Geometry check sheet. Reference: the model listing, model coordinates, mm. A direction names the side the tool comes from. Give positions to 0.01 mm unless a question says otherwise; leave off trailing zeros. Write each loop counter-clockwise with the first axis right and the second up, starting at its lowest first coordinate (ties: lowest second). Pieces come first, ordered by that corner, then holes. Notation, with made-up numbers: (58.25, -18.75) - (75.25, -18.75) arc R33 cw to (75.25, 19.25) - close; hole circle Ø1 at (-14.75, 24.5). An arc over 180 degrees is marked (long way). Write item = value, one per line. Start each with the question number.
(1) Thickness scan on L1, parallel to X at y = -45.5, z = 22; L2, parallel to Y at x = 25, z = 57. Record the ranges inside material, lowest first.
(2) Section check D-D, the plane z = 53. Enter the section's corners in (x, y), plus the area to 3 significant figures.
(3) Section check B-B, the plane x = -56. Enter the section's corners in (y, z).
(4) Depth check by flat-ended pin: pin 1 Ø12 at (x, y) = (14.5, -46.5) entering from -Z; pin 2 Ø5.5 at (y, z) = (-15.96, 19.23) entering from -X; pin 3 Ø6.5 at (x, z) = (33.28, 79.04) entering from +Y. Enter the tip coordinate at first touch or a pass-through.
(5) Draft check along Y on faces 1 (the flat face through (-5, -51.506, 41)), 2 (the cylindrical face through (60.6, -16.47, 61.35)), 3 (the flat face through (63.102, -26, 41)). Enter one of: pulls with the +Y half, pulls with the -Y half, needs draft (parallel to the pull), parting line crosses it, or undercut.
(6) Section check A-A, the plane z = 35. Enter the section's corners in (x, y).
(7) Section check C-C, the plane y = -23. Enter the section's corners in (x, z), plus the area to 3 significant figures.
(8) Access from +Z, -Z, +X, -X, +Y, -Y to the whole of each face (thin tool, end or side, straight path). Record for faces 4 (the flat face through (58.022, -4, 41)), 5 (the flat face through (-68.978, -54, 41)).
```python
from build123d import *

# Parameters (mm, degrees)
F1_DEPTH = 82.55
F3_D     = 19.05
F4_D     = 4.7752
F5_D     = 4.7752
F7_D     = 5.08


with BuildPart() as f1:
    # F0 (on Top) → F1 (new body)
    with BuildSketch(Plane.XY):
        Polygon((58.022249, -51.505502), (-68.977751, -51.505502), (-68.977751, -56.585502), (63.102249, -56.585502), (63.102249, 24.694498), (58.022249, 24.694498), align=None)
    extrude(amount=F1_DEPTH)

    # F3 (through all)
    with Locations(Plane(origin=(58.022249, 0, 0), x_dir=(0, -1, 0), z_dir=(-1, 0, 0))):
        with Locations((15.955091, 41.455898)):
            Hole(F3_D / 2)

    # F4 (through all)
    with Locations(Plane(origin=(58.022249, 0, 0), x_dir=(0, -1, 0), z_dir=(-1, 0, 0))):
        with Locations((15.955091, 63.680898)):
            Hole(F4_D / 2)

    # F5 (through all)
    with Locations(Plane(origin=(58.022249, 0, 0), x_dir=(0, -1, 0), z_dir=(-1, 0, 0))):
        with Locations((15.955091, 19.230898)):
            Hole(F5_D / 2)

    # F7 (through all)
    with Locations(Plane(origin=(0, -51.505502, 0), x_dir=(-1, 0, 0), z_dir=(0, 1, 0))):
        with Locations((-33.277512, 79.039508), (54.963514, 79.039508), (54.963514, 3.499908), (-33.277512, 3.499908)):
            Hole(F7_D / 2)


solid = f1.part
```
Model answer:
q1.L1 = 58.02 to 63.1
q1.L2 = -56.59 to -51.51
q2.outline = (-68.98, -56.59) - (63.1, -56.59) - (63.1, 24.69) - (58.02, 24.69) - (58.02, -51.51) - (-68.98, -51.51) - close
q2.area = 1,060 mm²
q3.outline = (-56.59, 0) - (-51.51, 0) - (-51.51, 1.18) - (-56.59, 1.18) - close; (-56.59, 5.82) - (-51.51, 5.82) - (-51.51, 76.72) - (-56.59, 76.72) - close; (-56.59, 81.36) - (-51.51, 81.36) - (-51.51, 82.55) - (-56.59, 82.55) - close
q4.pin_1 = 0
q4.pin_2 = 58.02
q4.pin_3 = -51.51
q5.face_1 = pulls with the +Y half
q5.face_2 = undercut
q5.face_3 = needs draft
q6.outline = (-68.98, -56.59) - (63.1, -56.59) - (63.1, -22.96) - (58.02, -22.96) - (58.02, -51.51) - (-68.98, -51.51) - close; (58.02, -8.95) - (63.1, -8.95) - (63.1, 24.69) - (58.02, 24.69) - close
q7.outline = (58.02, 0) - (63.1, 0) - (63.1, 35.05) - (58.02, 35.05) - close; (58.02, 47.87) - (63.1, 47.87) - (63.1, 82.55) - (58.02, 82.55) - close
q7.area = 354 mm²
q8.face_4 = +Z, -Z, -X, +Y
q8.face_5 = +Z, -Z, -X, +Y, -Y
